Check sheet for the modelled part. Datum: model origin and axes. Units: mm. A direction names the side the tool comes from. Round coordinates to 2 decimals unless told otherwise and drop trailing zeros. Write each loop counter-clockwise with the first axis right and the second up, starting at its lowest first coordinate (ties: lowest second). Pieces come first, ordered by that corner, then holes. Notation, with made-up numbers: (53.5, 68) -> (59.5, 68) arc R34 cw to (59.5, 104) -> close; hole circle Ø7 at (25.25, 10.25). An arc over 180 degrees is marked (long way). Write item = value, one per line.
Autodesk Inventor part; units mm, degrees
ref_plane "YZ Plane" through (0, 0, 0) normal (1, 0, 0) x (0, 1, 0)
ref_plane "XZ Plane" through (0, 0, 0) normal (0, 1, 0) x (-1, 0, 0)
ref_plane "XY Plane" through (0, 0, 0) normal (0, 0, 1) x (1, 0, 0)
sketch "Sketch1" plane through (0, 0, 0) normal (0, 0, 1) x (1, 0, 0)
  arc A0 (-97, -1740) -> (-70, 0) centre (-11100.8726, -699.0408) ccw
  line L0 (0, 0) -> (-70, 0)
  line L1 (0, -16.732) -> (-68.9524, -16.732) construction
  line L2 (0, -496.732) -> (-49.7243, -496.732) construction
  line L3 (0, -976.732) -> (-51.3615, -976.732) construction
  line L4 (0, -1456.732) -> (-73.8734, -1456.732) construction
  line L5 (-97, -1740) -> (0, -1740)
  line L6 (0, 0) -> (0, -1740)
  line L7 (0, -1730) -> (-10.3553, -1740)
  point P0 (-20, 0)
  dimension "d33" = 50
  dimension "d58" = 480
  dimension "d59" = 480
  dimension "d60" = 480
  dimension "d141" = 1740
  dimension "d148" = 70
  dimension "d149" = 11053
  dimension "d150" = 97
  dimension "d151" = 136
  dimension "d153" = 10
extrude "Plate3" add sketch "Sketch1" along normal blind 3 contours A0 L0 L6 L7 L5
sketch "Sketch3" plane through (-3, 0, 3) normal (1, 0, 0) x (0, 1, 0)
  line L0 (-1730, 0) -> (0, 0)
  line L1 (0, 0) -> (0, 20)
  line L2 (0, 20) -> (-1730, 20)
  line L3 (-1730, 20) -> (-1730, 0)
edge flange "Flange2" height 20 angle 90 thickness 3 bend radius 5 thickness toward (1, 0, 0) relief round relief width 3 relief depth 1.5 edges at (0, -865, 3) wall of the first edge with corners at (-3, -1730, 3) (-3, 0, 3) (-3, 0, -17) (-3, -1730, -17)
bend "Bend2"
corner "Corner2"
sketch "Sketch5" plane through (0, 0, 0) normal (0, 0, 1) x (1, 0, 0)
  line L0 (-8, -1737.7255) -> (-8, 0)
  line L1 (-70, 0) -> (-8, 0)
  arc A0 (-97, -1740) -> (-70, 0) centre (-11100.8726, -699.0408) ccw
  line L2 (0, 0) -> (0, -1730)
  line L3 (0, -198.9) -> (-28, -198.9)
  line L4 (0, -201.1) -> (-3, -201.1)
  line L5 (-3, -1730) -> (-3, 0)
  line L6 (-28, -198.9) -> (-28, -201.1)
  line L7 (0, -608.9) -> (-48.2402, -608.9) construction
  line L8 (0, -1018.9) -> (-52.5018, -1018.9) construction
  line L9 (0, -1428.9) -> (-71.9962, -1428.9) construction
  line L10 (-10.3553, -1740) -> (-97, -1740)
  line L11 (0, -198.9) -> (0, -218.9)
  line L12 (-3, -198.9) -> (-3, -201.1) construction
  line L13 (0, -218.9) -> (-3, -218.9)
  line L14 (-28, -198.9) -> (-59.1939, -198.9) construction
  line L15 (-28, -201.1) -> (-59.0945, -201.1) construction
  line L16 (-3, -201.1) -> (-3, -218.9)
  line L17 (-3, -201.1) -> (-28, -201.1)
  line L18 (-3, -218.9) -> (-8, -218.9)
  line L19 (-8, -1737.7255) -> (-10.3553, -1740)
  line L20 (-4.4351, -201.1) -> (0, -205.5351)
  line L21 (-4.4351, -201.1) -> (1.8371, -201.1) construction
  line L22 (-10.3553, -1740) -> (-10.3553, -1770)
  point P0 (0, 0)
  point P1 (845.25, -380.4205)
  point P2 (848, -380.4205)
  point P3 (-28, -200)
  point P4 (850, -410.4205)
  point P5 (-3, -198.9)
  point P6 (-3, -218.9)
  point P7 (-8, -201.1)
  point P8 (0, -205.5351)
  dimension "d69" = 1730
  dimension "d70" = 2.2
  dimension "d76" = 59.1939
  dimension "d80" = 48.2402
  dimension "d102" = 71.9962
  dimension "d104" = 52.5018
  dimension "d106" = 3
  dimension "d107" = 20
  dimension "d108" = 200
  dimension "d112" = 28
  dimension "d142" = 410
  dimension "d143" = 410
  dimension "d144" = 410
  dimension "d154" = 45
  dimension "d155" = 30
  dimension "d156" = 341.1
extrude "Extrusion2" cut sketch "Sketch5" along normal through all both and the other way through all contours L17 L6 L3 L0 | L0 L3 L5 L17 | L17 L5 L20 | L5 L4 L2 L20 | L3 L2 L4 L5
pattern_linear "Rectangular Pattern3" count 4 spacing 410 along (0, -1, 0) of "Extrusion2"
sketch "Sketch7" plane through (0, 0, 0) normal (0, 0, 1) x (1, 0, 0)
  line L0 (0, 0) -> (0, -198.9)
  line L1 (0, 0) -> (-100, 0)
  line L2 (-100, 0) -> (-100, -520)
  line L3 (-100, -520) -> (0, -520)
  line L4 (0, -520) -> (0, 0)
  line L5 (-100, -1740) -> (0, -1740)
  line L6 (0, -1740) -> (0, -520)
  line L7 (0, -520) -> (-100, -520)
  line L8 (-100, -520) -> (-100, -1740)
  line L9 (-97, -1740) -> (-10.3553, -1740)
  point P0 (-50, -1740)
  dimension "d157" = 100
  dimension "d158" = 520
extrude "Extrusion3" cut sketch "Sketch7" along normal through all both and the other way through all contours L6 L5 L8 L3
equation "\"БОРТ_стрингер_3_высота\" = 59"
equation "\"БОРТ_стрингер_4_высота\" = 48"
equation "\"БОРТ_стрингер_5_высота\" = 53"
equation "\"БОРТ_стрингер_6_высота\" = 72"
properties part number "MSC 348 RIB BOARD" material "Stainless Steel"
(1) Sectioned sample at A-A on z = -11. Enter the section's corners in (x, y).
Worked answers:
outline = (-3, -520) -> (0, -520) -> (0, -205.54) -> (-3, -202.54) -> close; (-3, -198.9) -> (0, -198.9) -> (0, 0) -> (-3, 0) -> close
(2) Sectioned sample at B-B on y = -446.5. Enter the section's corners in (x, z).
Worked answers:
outline = (-50.76, 0) -> (-8, 0) arc R5 cw to (-3, -5) -> (-3, -17) -> (0, -17) -> (0, -5) arc R8 ccw to (-8, 3) -> (-50.76, 3) -> close
(3) Access from +Z, -Z, +X, -X, +Y, -Y to the whole of each face (thin tool, end or side, straight path). Record for faces 1 (the flat face through (-3, -101, -11)), 2 (the cylindrical face through (-2.281, -100.842, 0.594)).
Worked answers:
face_1 = -Z, -X, +Y, -Y
face_2 = +Z, +X, +Y, -Y
(4) Sectioned sample at D-D on y = -148. Enter the section's corners in (x, z).
Worked answers:
outline = (-61.62, 0) -> (-8, 0) arc R5 cw to (-3, -5) -> (-3, -17) -> (0, -17) -> (0, -5) arc R8 ccw to (-8, 3) -> (-61.62, 3) -> close
(5) Sectioned sample at C-C on x = -44. Enter the section's corners in (y, z).
Worked answers:
outline = (-520, 0) -> (0, 0) -> (0, 3) -> (-520, 3) -> close
(6) Go/stop test with flat-tipped pins: P1, Ø6, axis at y = -69, z = -11, coming from the -X side; P2, Ø4, axis at x = -46, z = -1.5, coming from the -Y side; P3, Ø10, axis at y = -353, z = -6.5, coming from the -X side; P4, Ø6, axis at x = -11, z = -3.5, coming from the -Y side. Record where each tip stops, or that it passes through.
Worked answers:
P1 = -3
P2 = -520
P3 = -4.43
P4 = through
(7) Material ranges on L1, parallel to X at y = -67, z = -12.25; L2, parallel to Z at x = -52, y = -336; L3, parallel to Z at x = -6, y = -410.5, recorded low to high. Write a range as [from, to].
Worked answers:
L1 = [-3, 0]
L2 = [0, 3]
L3 = [-0.42, 2.75]
(8) Release check for a two-part mould opening along Y. For faces 3 (the flat face through (-9.8, -198.9, 0.4)), 4 (the flat face through (-19.3, -520, 0.4)), 5 (the flat face through (-3, -363, -11)), 6 (the flat face through (-29.7, 0, 0.4)) record: pulls with the +Y half, pulls with the -Y half, needs draft (parallel to the pull), parting line crosses it, or undercut.
Worked answers:
face_3 = undercut
face_4 = pulls with the -Y half
face_5 = needs draft
face_6 = pulls with the +Y half
